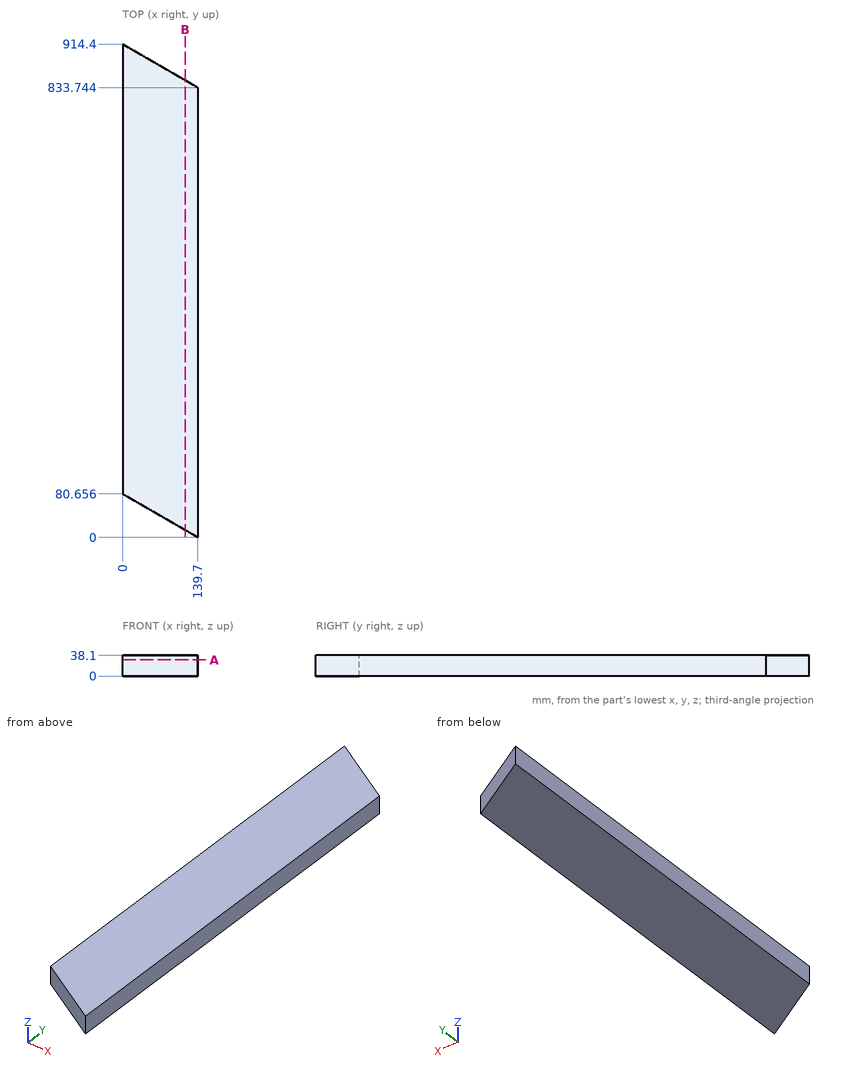
Verification items for this drawing (mm, ordinates from the low corner). Give positions to 0.01 mm unless a question says otherwise; leave off trailing zeros. Write each loop counter-clockwise with the first axis right and the second up, starting at its lowest first coordinate (ties: lowest second). Pieces come first, ordered by that corner, then holes. Notation, with made-up numbers: (-24.5, -29.75) -> (-10.5, -29.75) arc R20 cw to (-10.5, 0.25) -> close; hole circle Ø9 at (40, 27). An arc over 180 degrees is marked (long way). Use CSV: the item, a comma, the result in double quotes. Start each with the question number.
Q1. Cross-section at B-B on x = 116. Enter the section's corners in (y, z), and give its area (3 significant figures).
Q2. Cross-section at A-A on z = 30. Enter the section's corners in (x, y).
Q3. Scan lines: line 1 along Y through (x, z) = (95, 21.5); line 2 along Y through (x, z) = (35, 23). Record each from-to range of solid material in increasing order.
Q4. Depth check by flat-ended pin: P1, Ø12, axis at x = 23, y = 312.5, coming from the -Z side; P2, Ø2, axis at x = 50, z = 30, coming from the +Y side; P3, Ø3, axis at x = 93.5, z = 30, coming from the -Y side; P4, Ø2, axis at x = 46, z = 18, coming from the +Y side. Enter the tip coordinate at first touch or a pass-through.
Working result:
1,outline,"(13.68, 0) -> (847.43, 0) -> (847.43, 38.1) -> (13.68, 38.1) -> close"
1,area,"31,800 mm^2"
2,outline,"(0, 80.66) -> (139.7, 0) -> (139.7, 833.74) -> (0, 914.4) -> close"
3,line 1,"y = 25.81 to 859.55"
3,line 2,"y = 60.45 to 894.19"
4,P1,"stops at z = 0"
4,P2,"stops at y = 886.11"
4,P3,"stops at y = 25.81"
4,P4,"stops at y = 888.42"
